from build123d import *

# Parameters (mm, degrees)
SKETCH1_W           = 64
SKETCH1_H           = 92
BOSS_EXTRUDE1_DEPTH = 3
SKETCH2_W           = 9.5
SKETCH2_H           = 12.5
CUT_EXTRUDE1_DEPTH  = 3
FILLET1_R           = 4.75
FILLET2_R           = 2
CUT_EXTRUDE2_START  = -10.454
SKETCH6_R           = 5.375
CUT_EXTRUDE2_DEPTH  = 10.454
SKETCH8_R           = 13.356098795
CUT_EXTRUDE3_DEPTH  = 3
FILLET3_R           = 2
FILLET4_R           = 2


# Some blends are built 0.0001 mm under size
with BuildPart() as part:
    # Sketch1 → Boss-Extrude1 (new body)
    with BuildSketch(Plane(origin=(0, 0, 0), x_dir=(1, 0, 0), z_dir=(0, 1, 0))):
        Rectangle(SKETCH1_W, SKETCH1_H)
    extrude(amount=BOSS_EXTRUDE1_DEPTH)

    # Sketch2 → Cut-Extrude1 (cut)
    with BuildSketch(Plane(origin=(0, 3, 0), x_dir=(1, 0, 0), z_dir=(0, 1, 0))):
        with Locations((22.25, 36.15)):
            Rectangle(SKETCH2_W, SKETCH2_H)
        with Locations((-22.25, 36.15)):
            Rectangle(SKETCH2_W, SKETCH2_H)
        with Locations((22.25, -36.15)):
            Rectangle(SKETCH2_W, SKETCH2_H)
        with Locations((-22.25, -36.15)):
            Rectangle(SKETCH2_W, SKETCH2_H)
    extrude(amount=-CUT_EXTRUDE1_DEPTH, mode=Mode.SUBTRACT)

    # Fillet1
    fillet1_edges = [part.edges().sort_by_distance(p)[0] for p in [
        (27, 1.5, 42.4),
        (17.5, 1.5, 42.4),
        (17.5, 1.5, 29.9),
        (27, 1.5, 29.9),
        (-27, 1.5, 42.4),
        (-17.5, 1.5, 42.4),
        (-17.5, 1.5, 29.9),
        (-27, 1.5, 29.9),
        (27, 1.5, -29.9),
        (17.5, 1.5, -29.9),
        (27, 1.5, -42.4),
        (17.5, 1.5, -42.4),
        (-17.5, 1.5, -29.9),
        (-27, 1.5, -29.9),
        (-17.5, 1.5, -42.4),
        (-27, 1.5, -42.4),
    ]]
    fillet(fillet1_edges, radius=FILLET1_R - 0.0001)  # a hair under: the kernel refuses the full size

    # Sketch5 → Revolve1 (revolve)
    with BuildSketch(Plane(origin=(0, 0, 0), x_dir=(0, 0, -1), z_dir=(1, 0, 0))):
        with BuildLine():
            Line((17.443, 3), (12.48, 5.785))
            Line((12.48, 5.785), (8.652, 6.959))
            ThreePointArc((8.652, 6.959), (7.100088069, 8.476564665), (6.205, 10.454))
            Line((6.205, 10.454), (0, 10.454))
            Line((0, 10.454), (0, 3))
            Line((0, 3), (2, 3))
            Line((2, 3), (2, 8.454))
            Line((2, 8.454), (4.805757283, 8.454))
            ThreePointArc((4.805757283, 8.454), (6.064441281, 6.572314424), (7.806379809, 5.126397352))
            Line((7.806379809, 5.126397352), (11.688413221, 3.935825977))
            Line((11.688413221, 3.935825977), (13.356098795, 3))
            Line((13.356098795, 3), (17.443, 3))
        make_face()
    revolve(axis=Axis((0, -11.842752106, 0), (0, 1, 0)))

    # Fillet2
    fillet2_edges = [part.edges().sort_by_distance(p)[0] for p in [
        (0, 5.785, 12.48),
    ]]
    fillet(fillet2_edges, radius=FILLET2_R)

    # Sketch6 → Cut-Extrude2 (cut)
    with BuildSketch(Plane(origin=(0, 10.454, 0), x_dir=(1, 0, 0), z_dir=(0, 1, 0)).offset(CUT_EXTRUDE2_START)):
        with Locations(Location((0, 0, 0), (0, 0, 270))):
            Circle(SKETCH6_R)
    extrude(amount=CUT_EXTRUDE2_DEPTH, mode=Mode.SUBTRACT)

    # Sketch8 → Cut-Extrude3 (cut)
    with BuildSketch(Plane(origin=(0, 0, 0), x_dir=(-1, 0, 0), z_dir=(0, -1, 0))):
        with Locations(Location((0, 0, 0), (0, 0, 90))):
            Circle(SKETCH8_R)
    extrude(amount=-CUT_EXTRUDE3_DEPTH, mode=Mode.SUBTRACT)

    # Fillet3
    fillet3_edges = [part.edges().sort_by_distance(p)[0] for p in [
        (0, 3, 13.356098795),
    ]]
    fillet(fillet3_edges, radius=FILLET3_R)

    # Fillet4
    # the kernel refuses this fillet: 2 mm, written as the material it takes off along each edge
    with BuildSketch(Plane(origin=(0, 0, 0), x_dir=(0, 0, -1), z_dir=(-1, 0, 0))) as fillet4_piece_1:
        with BuildLine():
            CenterArc((15.352435599, -2), FILLET4_R, 90, 87.54885706)
            Line((15.352435599, 0), (15.352435599, 0.2))
            Line((15.352435599, 0.2), (13.356098795, 0.2))
            Line((13.356098795, 0.2), (13.156098795, 0))
            ThreePointArc((13.156098795, 0), (13.156095386, -1.828930112), (13.154448481, -1.905911573))
            Line((13.154448481, -1.905911573), (13.354265492, -1.914465067))
        make_face()
    revolve(axis=Axis((0, 0, 0), (0, -1, 0)), mode=Mode.SUBTRACT)


solid = part.part
Geometry check sheet. Reference: the model listing, model coordinates, mm. A direction names the side the tool comes from. Coordinates: 2 decimals unless noted, no trailing zeros. Order: outer loops, then holes, each group sorted by start corner. A loop starts at its lowest first (then second) coordinate and runs counter-clockwise, first axis right, second up. Notation, with made-up numbers: (57.5, -39) -> (81.5, -39) arc R12 cw to (81.5, -19) -> close; hole circle Ø3 at (46.25, 37.5). An arc over 180 degrees is marked (long way). Use a Markdown table: item, result. Add a question column.
1. Go/stop test with flat-tipped pins: pin 1 Ø1.5 at (x, y) = (3.5, 9) entering from -Z; pin 2 Ø4 at (y, z) = (7.5, -9) entering from +X (3 decimals). Record where each tip stops, or that it passes through.
2. Material ranges on L1, parallel to Z at x = -26, y = 0.75; L2, parallel to Y at x = 4, z = -34.5; L3, parallel to X at y = 8.85, z = 0 (3 decimals), recorded low to high.
3. Cross-section at B-B (x = -20). Enter the section's corners in (y, z).
4. Mould release check, pull along Z, two halves, no side actions. Record for faces 1 (the face through (-15, 3, 10)), 2 (the face through (8.618, 6.905, 1.914)), 3 (the face through (-18.928, 1.479, 41.046)), 4 (the face through (3.633, 8.934, -3.962)): pulls with the +Z half, pulls with the -Z half, needs draft (parallel to the pull), parting line crosses it, or undercut.
5. Cross-section at A-A (z = -36). Enter the section's corners in (x, y), and give its area (3 significant figures).
6. Set-up check for faces 5 (the face through (18.928, 1.479, -31.254)), 6 (the face through (32, 1, 1)): record each of +Z, -Z, +X, -X, +Y, -Y from which the full face is reachable in a straight line by a thin tool's end or side.
Filled sheet:
| question | item | result |
|---|---|---|
| 1 | pin 1 | z = -6.48 |
| 1 | pin 2 | x = 9.695 |
| 2 | L1 | -46 to -40.57, -31.73 to 31.73, 40.57 to 46 |
| 2 | L2 | 0 to 3 |
| 2 | L3 | -6.859 to -5.375, 5.375 to 6.859 |
| 3 | outline | (0, -46) -> (3, -46) -> (3, -41.83) -> (0, -41.83) -> close; (0, -30.47) -> (3, -30.47) -> (3, 30.47) -> (0, 30.47) -> close; (0, 41.83) -> (3, 41.83) -> (3, 46) -> (0, 46) -> close |
| 4 | face 1 | needs draft |
| 4 | face 2 | parting line crosses it |
| 4 | face 3 | undercut |
| 4 | face 4 | undercut |
| 5 | outline | (-32, 0) -> (-27, 0) -> (-27, 3) -> (-32, 3) -> close; (-17.5, 0) -> (17.5, 0) -> (17.5, 3) -> (-17.5, 3) -> close; (27, 0) -> (32, 0) -> (32, 3) -> (27, 3) -> close |
| 5 | area | 135 mm2 |
| 6 | face 5 | +Y, -Y |
| 6 | face 6 | +Z, -Z, +X, +Y, -Y |
